```python
from build123d import *

# Parameters (mm, degrees)
BOSS_EXTRUDE1_DEPTH = 2
SKETCH3_R           = 4
SKETCH3_R_2         = 2
BOSS_EXTRUDE2_DEPTH = 5


with BuildPart() as part:
    # Sketch2 → Boss-Extrude1 (new body)
    with BuildSketch(Plane.XY):
        with BuildLine():
            Line((0.171455577, 3.939749203), (44.786956522, 1.998108747))
            ThreePointArc((44.786956522, 1.998108747), (46.7, 0), (44.786956522, -1.998108747))
            Line((44.786956522, -1.998108747), (0.171455577, -3.939749203))
            ThreePointArc((0.171455577, -3.939749203), (-3.943478261, 0), (0.171455577, 3.939749203))
        make_face()
    extrude(amount=BOSS_EXTRUDE1_DEPTH)

    # Sketch3 → Boss-Extrude2 (add)
    with BuildSketch(Plane.XY.offset(2)):
        with Locations(Location((0, 0, 0), (0, 0, 282.135260603))):
            Circle(SKETCH3_R)
        with Locations(Location((44.7, 0, 0), (0, 0, 272.491906369))):
            Circle(SKETCH3_R_2)
    extrude(amount=BOSS_EXTRUDE2_DEPTH)


solid = part.part
```
CAD build for the part. Positions are in the model's coordinates, mm. Coordinates: 2 decimals unless noted, no trailing zeros. Order: outer loops, then holes, each group sorted by start corner. A loop starts at its lowest first (then second) coordinate and runs counter-clockwise, first axis right, second up. Notation, with made-up numbers: M -0.5,-33.5 L 46.5,-33.5 A18 ccw 46.5,-14.5 Z; hole C 15.25,4 d2. An arc over 180 degrees is marked long. Write each question's results on one line, items separated by ' | '. Start each with the question number.
Q1. Drill centre lines: probe 1 along X at (y, z) = (0, 3.25); probe 2 along Z at (x, y) = (32, -2.25); probe 3 along X at (y, z) = (1.5, 3.75). Where is each one in solid material? Low to high. Write a range as from..to.
Q2. Pull direction X, two halves, no side cores. Call faces 1 (the flat face through (22.792, -2.955, 0.986)), 2 (the cylindrical face through (-0.721, -3.934, 4.465)), 3 (the flat face through (0, 0, 7)): +X half, -X half, draft (parallel to the pull), parting line (faces both ways), or undercut.
Q3. Cut at D-D (y = 3.25). List the corners of the cut face in (x, z).
Q4. Cut at A-A (z = 4). List the corners of the cut face in (x, y).
Q5. Cut at C-C (x = 2). List the corners of the cut face in (y, z).
Q6. Cut at B-B (y = 0). List the corners of the cut face in (x, z).
Found:
1) probe 1: -4..4, 42.7..46.7 | probe 2: 0..2 | probe 3: -3.71..3.71, 43.38..46.02
2) face 1: +X half | face 2: undercut | face 3: draft
3) outline: M -2.33,2 L -2.23,2 L -2.23,0 L 16.02,0 L 16.02,2 L 2.33,2 L 2.33,7 L -2.33,7 Z
4) outline: C 0,0 d8; C 44.7,0 d4
5) outline: M -3.86,0 L 3.86,0 L 3.86,2 L 3.46,2 L 3.46,7 L -3.46,7 L -3.46,2 L -3.86,2 Z
6) outline: M -4,2 L -3.94,2 L -3.94,0 L 46.7,0 L 46.7,7 L 42.7,7 L 42.7,2 L 4,2 L 4,7 L -4,7 Z
